from build123d import *

# Parameters (mm, degrees)
SM_BASE_FLANGE_1_DEPTH = 50
SKETCH_3_R             = 6.9
CUT_EXTRUDE_2_DEPTH    = 10
SKETCH_4_R             = 6.5
CUT_EXTRUDE_3_DEPTH    = 10
OTHER_START            = 49.143921292
OTHER_1_OUTLINE_W      = 8
OTHER_1_OUTLINE_H      = 38
OTHER_1_DEPTH          = 3.535533906
OTHER_START_2          = 84.499260352
OTHER_1_2_OUTLINE_W    = 8
OTHER_1_2_OUTLINE_H    = 10
OTHER_1_2_DEPTH        = 3.535533906
OTHER_START_3          = -3.535533906
OTHER_1_3_OUTLINE_W    = 10
OTHER_1_3_OUTLINE_H    = 7
OTHER_1_3_DEPTH        = 3.535533906
OTHER_START_4          = 31.819805153
OTHER_1_4_OUTLINE_W    = 38
OTHER_1_4_OUTLINE_H    = 7
OTHER_1_4_DEPTH        = 3.535533906


# Read off the part's stored shape, not the designer's step: Затупленный угол1
# Sheet-metal steps are written as plain solids
with BuildPart() as part:
    # Sketch 1 → Базовая кромка1 (new body)
    with BuildSketch(Plane.XY):
        with BuildLine():
            Line((-391.45, 74.5), (-391.45, 10))
            ThreePointArc((-391.45, 10), (-388.521067812, 2.928932188), (-381.45, 0))
            Line((-381.45, 0), (0, 0))
            Line((0, 0), (0, 5))
            Line((0, 5), (-381.45, 5))
            ThreePointArc((-381.45, 5), (-384.985533906, 6.464466094), (-386.45, 10))
            Line((-386.45, 10), (-386.45, 74.5))
            Line((-386.45, 74.5), (-391.45, 74.5))
        make_face()
    extrude(amount=SM_BASE_FLANGE_1_DEPTH)

    # Эскиз3 → Вырез-Вытянуть2 (cut)
    with BuildSketch(Plane(origin=(0, 5, 0), x_dir=(1, 0, 0), z_dir=(0, 1, 0))):
        with Locations(Location((-17.5, -25, 0), (0, 0, 270))):
            Circle(SKETCH_3_R)
    extrude(amount=-CUT_EXTRUDE_2_DEPTH, mode=Mode.SUBTRACT)

    # Эскиз4 → Вырез-Вытянуть3 (cut)
    with BuildSketch(Plane.ZY.offset(391.45)):
        with BuildLine():
            Line((31.5, 32), (31.5, 35.5))
            ThreePointArc((31.5, 35.5), (25, 29), (18.5, 35.5))
            Line((18.5, 35.5), (18.5, 32))
            ThreePointArc((18.5, 32), (25, 25.5), (31.5, 32))
        make_face()
        with Locations((25, 35.5)):
            Circle(SKETCH_4_R)
        with BuildLine():
            Line((31.5, 35.5), (31.5, 39))
            ThreePointArc((31.5, 39), (25, 45.5), (18.5, 39))
            Line((18.5, 39), (18.5, 35.5))
            ThreePointArc((18.5, 35.5), (25, 42), (31.5, 35.5))
        make_face()
        with BuildLine():
            Line((31.5, 57), (31.5, 60.5))
            ThreePointArc((31.5, 60.5), (25, 54), (18.5, 60.5))
            Line((18.5, 60.5), (18.5, 57))
            ThreePointArc((18.5, 57), (25, 50.5), (31.5, 57))
        make_face()
        with Locations((25, 60.5)):
            Circle(SKETCH_4_R)
        with BuildLine():
            Line((31.5, 60.5), (31.5, 64))
            ThreePointArc((31.5, 64), (25, 70.5), (18.5, 64))
            Line((18.5, 64), (18.5, 60.5))
            ThreePointArc((18.5, 60.5), (25, 67), (31.5, 60.5))
        make_face()
    extrude(amount=-CUT_EXTRUDE_3_DEPTH, mode=Mode.SUBTRACT)

    # Other 1 outline → Other 1 (cut)
    with BuildSketch(Plane(origin=(0, 0, 0), x_dir=(1, 0, 0), z_dir=(0, 0.7071067811865476, -0.7071067811865476)).offset(OTHER_START)):
        with Locations((-389, -67)):
            Rectangle(OTHER_1_OUTLINE_W, OTHER_1_OUTLINE_H)
    extrude(amount=OTHER_1_DEPTH, mode=Mode.SUBTRACT)

    # Other 1 2 outline → Other 1 2 (cut)
    with BuildSketch(Plane(origin=(0, 0, 0), x_dir=(1, 0, 0), z_dir=(0, 0.7071067811865476, 0.7071067811865476)).offset(OTHER_START_2)):
        with Locations((-389, 17)):
            Rectangle(OTHER_1_2_OUTLINE_W, OTHER_1_2_OUTLINE_H)
    extrude(amount=OTHER_1_2_DEPTH, mode=Mode.SUBTRACT)

    # Other 1 3 outline → Other 1 3 (cut)
    with BuildSketch(Plane(origin=(0, 0, 0), x_dir=(0.707106781186549, 0, 0.707106781186546), z_dir=(0.707106781186546, 0, -0.707106781186549)).offset(OTHER_START_3)):
        with Locations((0, -2.5)):
            Rectangle(OTHER_1_3_OUTLINE_W, OTHER_1_3_OUTLINE_H)
    extrude(amount=OTHER_1_3_DEPTH, mode=Mode.SUBTRACT)

    # Other 1 4 outline → Other 1 4 (cut)
    with BuildSketch(Plane(origin=(0, 0, 0), x_dir=(0.707106781186549, 0, -0.707106781186546), z_dir=(0.707106781186546, 0, 0.707106781186549)).offset(OTHER_START_4)):
        with Locations((-21, 2.5)):
            Rectangle(OTHER_1_4_OUTLINE_W, OTHER_1_4_OUTLINE_H)
    extrude(amount=OTHER_1_4_DEPTH, mode=Mode.SUBTRACT)


solid = part.part
Can you work these out from the model? Positions are in its coordinate system, mm. A direction names the side the tool comes from. Coordinates: 2 decimals unless noted, no trailing zeros. Write each loop counter-clockwise with the first axis right and the second up, starting at its lowest first coordinate (ties: lowest second). Pieces come first, ordered by that corner, then holes. Notation, with made-up numbers: M 86.25,40.25 L 139.25,40.25 A17 ccw 139.25,61.25 Z; hole C 35,89 d3. An arc over 180 degrees is marked long. Use one line per item in the form item = value.
Q1. If we section it at C-C (x = -267): Write out the boundary of the cut face in (y, z), then the cut area to 3 significant figures.
Model answer:
outline = M 0,0 L 5,0 L 5,50 L 0,50 Z
area = 250 mm^2
Q2. I need wall thicknesses on line 1 along Z through (x, y) = (-17, 1); line 2 along Y through (x, z) = (-147, 17); line 3 along X through (y, z) = (38.5, 37). Which ranges of each line are inside material? Lowest first, please. Write a range as from..to.
Model answer:
line_1 = 0..18.12, 31.88..50
line_2 = 0..5
line_3 = -391.45..-386.45
Q3. For P1, Ø8.5, axis at x = -17.5, z = 25, coming from the +Y side; P2, Ø15, axis at x = -194.5, z = 35, coming from the +Y side; P3, Ø25, axis at y = 54, z = 22.5, coming from the +X side, each with a flat end and sliding along its axis, tell me the tip position at first contact or that it passes through.
Model answer:
P1 = through
P2 = 5
P3 = -386.45
Q4. If we section it at A-A (z = 25): Write out the boundary of the cut face in (x, y).
Model answer:
outline = M -391.45,10 A10 ccw -381.45,0 L -24.4,0 L -24.4,5 L -381.45,5 A5 cw -386.45,10 L -386.45,25.5 L -391.45,25.5 Z; M -391.45,45.5 L -386.45,45.5 L -386.45,50.5 L -391.45,50.5 Z; M -391.45,70.5 L -386.45,70.5 L -386.45,74.5 L -391.45,74.5 Z; M -10.6,0 L 0,0 L 0,5 L -10.6,5 Z
Q5. We'd pull the mould along Y, two halves only. Please class faces 4 (the flat face through (-199, 4, 0)), 5 (the cylindrical face through (-389, 45.5, 25.1)), 6 (the cylindrical face through (-388.6, 3.01, 24.65)): +Y half, -Y half, draft (parallel to the pull), parting line (faces both ways), or undercut.
Model answer:
face_4 = draft
face_5 = undercut
face_6 = -Y half
Q6. For faces 1 (the cylindrical face through (-389, 70.5, 25.1)), 2 (the flat face through (-188, 5, 25)), 3 (the flat face through (-193, 0, 25)), which set-ups out of +Z, -Z, +X, -X, +Y, -Y let a thin tool reach every point of the face, with its end or its side?
Model answer:
face_1 = +X, -X
face_2 = +Z, -Z, +X, +Y
face_3 = +Z, -Z, +X, -X, -Y
Q7. If we section it at B-B (z = 40): Write out the boundary of the cut face in (x, y).
Model answer:
outline = M -391.45,10 A10 ccw -381.45,0 L 0,0 L 0,5 L -381.45,5 A5 cw -386.45,10 L -386.45,74.5 L -391.45,74.5 Z
